Here's how the part is built. I have some questions about the finished solid (model axes, mm). A direction names the side the tool comes from. Round coordinates to 2 decimals unless told otherwise and drop trailing zeros. Write each loop counter-clockwise with the first axis right and the second up, starting at its lowest first coordinate (ties: lowest second). Pieces come first, ordered by that corner, then holes. Notation, with made-up numbers: (-28, -28.75) - (1, -28.75) arc R18 ccw to (1, -0.75) - close; hole circle Ø2 at (-8.75, 56.25). An arc over 180 degrees is marked (long way). Use one line per item in the form item = value. Start each with the question number.
1. If I drill on line 1 along Z through (x, y) = (-71.5, 2.75); line 2 along Z through (x, y) = (-76, 1.35); line 3 along X through (y, z) = (2.45, -162.5), over which ranges is the centre line in solid material (lowest first)?
2. Will these pins go through, and if not, where does the flat tip stop? pin 1 (1.6 mm diameter, centred on y = 3.5, z = 130, fed in from +X); pin 2 (1.2 mm diameter, centred on y = 2.5, z = 130.5, fed in from -X); pin 3 (2 mm diameter, centred on y = 2, z = -174.5, fed in from +X); pin 4 (6.5 mm diameter, centred on x = -73.82, z = 155.52, fed in from -Y).
3. Which directions (+Z, -Z, +X, -X, +Y, -Y) give clear straight access to the entire face, cutting with the end or side of a thin tool? Please do faces 1 (the flat face through (19, 5.63, 60)), 2 (the flat face through (-151.255, 2.776, -116.569)).
4. We'd pull the mould along X, two halves only. Please class faces 3 (the cylindrical face through (-38.68, 2.78, 126.08)), 4 (the flat face through (-159.833, 2.776, 88.291)), 5 (the cylindrical face through (-73.56, 2.854, -218.606)): +X half, -X half, draft (parallel to the pull), parting line (faces both ways), or undercut.
5. I want a section at B-B, the plane x = 52.5. List the corners of the cut face in (y, z) for me.
6. I want a section at C-C, the plane y = 2.3. State how many separate pieces and enclosed holes the cut face has, plus the area to 3 significant figures.
7. I want a section at A-A, the plane z = -58. List the corners of the cut face in (x, y) for me, plus the area to 3 significant figures.
```python
from build123d import *

# Parameters (mm, degrees)
SKETCH1_R           = 4
BOSS_EXTRUDE1_DEPTH = 5.63
FILLET1_R           = 20
FILLET2_R           = 20
FILLET3_R           = 10


with BuildPart() as part:
    # Sketch1 → Boss-Extrude1 (new body)
    with BuildSketch(Plane(origin=(0, 0, 0), x_dir=(1, 0, 0), z_dir=(0, 1, 0))):
        Polygon((-73.819651424, -202.975693425), (89.274098576, 14.482639908), (-73.819651424, 231.940973242), (-236.913401424, 14.482639908), align=None)
        with Locations(Location((-73.819651424, -155.517360092, 0), (0, 0, 270))):
            Circle(SKETCH1_R, mode=Mode.SUBTRACT)
        with BuildLine():
            Line((-214.413401424, 14.482639908), (-114.584807136, -118.622152475))
            ThreePointArc((-114.584807136, -118.622152475), (-109.396341366, -125.717430875), (-101.569651424, -129.718190449))
            Line((-101.569651424, -129.718190449), (-101.569651424, -131.218190449))
            Line((-101.569651424, -131.218190449), (-92.569651424, -131.218190449))
            Line((-92.569651424, -131.218190449), (-92.569651424, -129.718190449))
            ThreePointArc((-92.569651424, -129.718190449), (-86.926275258, -127.32463745), (-82.338731561, -123.258775507))
            Line((-82.338731561, -123.258775507), (-65.300571287, -123.258775507))
            ThreePointArc((-65.300571287, -123.258775507), (-60.71302759, -127.32463745), (-55.069651424, -129.718190449))
            Line((-55.069651424, -129.718190449), (-55.069651424, -131.218190449))
            Line((-55.069651424, -131.218190449), (-46.069651424, -131.218190449))
            Line((-46.069651424, -131.218190449), (-46.069651424, -129.718190449))
            ThreePointArc((-46.069651424, -129.718190449), (-38.242961482, -125.717430875), (-33.054495712, -118.622152475))
            Line((-33.054495712, -118.622152475), (66.774098576, 14.482639908))
            Line((66.774098576, 14.482639908), (-73.819651424, 201.940973242))
            Line((-73.819651424, 201.940973242), (-214.413401424, 14.482639908))
        make_face(mode=Mode.SUBTRACT)
        Polygon((-156.089651424, -81.157360092), (-153.329651424, -79.087360092), (-143.909651424, -91.647360092), (-146.669651424, -93.717360092), align=None, mode=Mode.SUBTRACT)
        Polygon((8.450348576, -81.157360092), (5.690348576, -79.087360092), (-3.729651424, -91.647360092), (-0.969651424, -93.717360092), align=None, mode=Mode.SUBTRACT)
        Polygon((-146.669651424, 122.682639908), (-155.969651424, 110.282639908), (-153.209651424, 108.212639908), (-143.909651424, 120.612639908), align=None, mode=Mode.SUBTRACT)
        Polygon((-0.969651424, 122.682639908), (8.330348576, 110.282639908), (5.570348576, 108.212639908), (-3.729651424, 120.612639908), align=None, mode=Mode.SUBTRACT)
    extrude(amount=BOSS_EXTRUDE1_DEPTH)

    # Fillet1
    fillet1_edges = [part.edges().sort_by_distance(p)[0] for p in [
        (89.274098576, 2.815, -14.482639908),
        (-73.819651424, 2.815, 202.975693425),
        (-236.913401424, 2.815, -14.482639908),
        (-73.819651424, 2.815, -231.940973242),
    ]]
    fillet(fillet1_edges, radius=FILLET1_R)

    # Fillet2
    fillet2_edges = [part.edges().sort_by_distance(p)[0] for p in [
        (66.774098576, 2.815, -14.482639908),
        (-73.819651424, 2.815, -201.940973242),
        (-214.413401424, 2.815, -14.482639908),
    ]]
    fillet(fillet2_edges, radius=FILLET2_R)

    # Fillet3
    fillet3_edges = [part.edges().sort_by_distance(p)[0] for p in [
        (-114.584807136, 2.815, 118.622152475),
        (-82.338731561, 2.815, 123.258775507),
        (-65.300571287, 2.815, 123.258775507),
        (-33.054495712, 2.815, 118.622152475),
    ]]
    fillet(fillet3_edges, radius=FILLET3_R)


solid = part.part
```
Model answer:
q1.line_1 = -218.47 to -188.47, 123.26 to 152.26, 158.78 to 189.51
q1.line_2 = -218.49 to -188.49, 123.26 to 152.16, 158.87 to 189.52
q1.line_3 = -125.9 to -103.4, -44.24 to -21.74
q2.pin_1 = -18.49
q2.pin_2 = -128.63
q2.pin_3 = -29.99
q2.pin_4 = through
q3.face_1 = +Z, -Z, +X, -X, +Y
q3.face_2 = +Y, -Y
q4.face_3 = undercut
q4.face_4 = -X half
q4.face_5 = parting line
q5.outline = (0, -63.51) - (5.63, -63.51) - (5.63, -33.51) - (0, -33.51) - close; (0, 4.55) - (5.63, 4.55) - (5.63, 34.55) - (0, 34.55) - close
q6.separate_pieces = 1
q6.enclosed_holes = 6
q6.area = 19,300 mm2
q7.outline = (-204.28, 0) - (-181.78, 0) - (-181.78, 5.63) - (-204.28, 5.63) - close; (34.14, 0) - (56.64, 0) - (56.64, 5.63) - (34.14, 5.63) - close
q7.area = 253 mm2
